Verification items for the finished model (mm, model axes). Give positions to 0.01 mm unless a question says otherwise; leave off trailing zeros. Loops run counter-clockwise (first coordinate to the right, second up) from the corner with the lowest first, then second, coordinate; pieces in that order, holes last. Notation, with made-up numbers: (-17.75, -24.75) - (33.25, -24.75) arc R37 ccw to (33.25, 14.25) - close; hole circle Ø9 at (-35, 27). An arc over 180 degrees is marked (long way). Use one line per item in the form item = value.
Solid Edge part; units mm, degrees
sketch "Sketch1" plane through (0, 0, 0) normal (0, -1, 0) x (1, 0, 0)
  circle A0 centre (0, 19.05) radius 0.762
  line L0 (-2.3495, 19.05) -> (-3.294, 0.5528)
  line L1 (2.3495, 19.05) -> (3.294, 0.5528)
  arc A1 (2.3495, 19.05) -> (-2.3495, 19.05) centre (0, 19.05) ccw
  arc A2 (-3.294, 0.5528) -> (3.294, 0.5528) centre (0, 0) ccw
  circle A3 centre (0, 0) radius 1.7526
extrude "Protrusion1" add sketch "Sketch1" along normal blind 1.524
properties material "Aluminum, 6061-T6"
1. Section check D-D, the plane x = 1. Record the cut outline in (y, z), then the cut area to 3 significant figures.
Result set:
outline = (-1.52, -3.19) - (0, -3.19) - (0, -1.44) - (-1.52, -1.44) - close; (-1.52, 1.44) - (0, 1.44) - (0, 21.18) - (-1.52, 21.18) - close
area = 32.7 mm²
2. Draft check along Z on faces 1 (the flat face through (0, -1.524, 9)), 2 (the cylindrical face through (1.67, -0.75, -0.53)), 3 (the flat face through (-2.815, -0.751, 9.931)). Enter one of: released by +Z, released by -Z, zero draft, split by the parting line, or undercut.
Result set:
face_1 = zero draft
face_2 = undercut
face_3 = released by +Z
3. Section check A-A, the plane x = 0. Record the cut outline in (y, z), then the cut area to 3 significant figures.
Result set:
outline = (-1.52, -3.34) - (0, -3.34) - (0, -1.75) - (-1.52, -1.75) - close; (-1.52, 1.75) - (0, 1.75) - (0, 18.29) - (-1.52, 18.29) - close; (-1.52, 19.81) - (0, 19.81) - (0, 21.4) - (-1.52, 21.4) - close
area = 30.0 mm²
4. Section check B-B, the plane z = 0. Record the cut outline in (x, y).
Result set:
outline = (-3.34, -1.52) - (-1.75, -1.52) - (-1.75, 0) - (-3.34, 0) - close; (1.75, -1.52) - (3.34, -1.52) - (3.34, 0) - (1.75, 0) - close
5. Scan lines: probe 1 along Z at (x, y) = (0, -0.55); probe 2 along Z at (x, y) = (0.5, -0.55); probe 3 along X at (y, z) = (-1.35, -0.5). Record each from-to range of solid material in increasing order.
Result set:
probe_1 = -3.34 to -1.75, 1.75 to 18.29, 19.81 to 21.4
probe_2 = -3.3 to -1.68, 1.68 to 18.47, 19.63 to 21.35
probe_3 = -3.3 to -1.68, 1.68 to 3.3
6. Section check C-C, the plane y = -0.4. Record the cut outline in (x, z).
Result set:
outline = (-3.29, 0.55) arc R3.34 ccw (long way) to (3.29, 0.55) - (2.35, 19.05) arc R2.35 ccw to (-2.35, 19.05) - close; hole circle Ø3.51 at (0, 0); hole circle Ø1.52 at (0, 19.05)
7. Depth check by flat-ended pin: pin 1 Ø4 at (x, z) = (0, 0) entering from -Y. Enter the tip coordinate at first touch or a pass-through.
Result set:
pin_1 = -1.52
